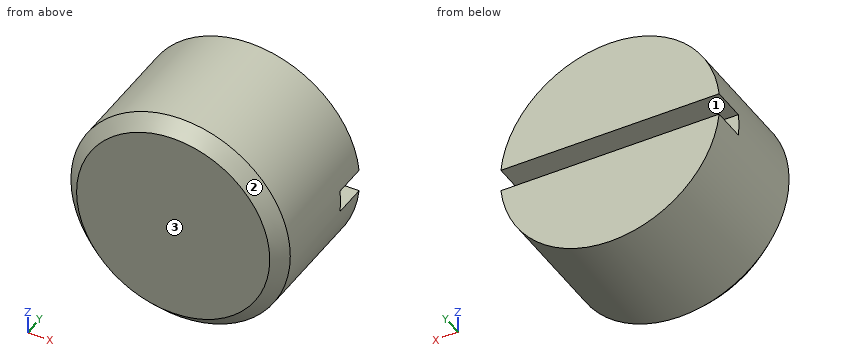
from build123d import *

# Parameters (mm, degrees)
SKETCH2_W          = 9.728
SKETCH2_H          = 1
CUT_EXTRUDE1_DEPTH = 1.5


with BuildPart() as part:
    # Sketch1 → Revolve1 (revolve)
    with BuildSketch(Plane.XY):
        Polygon((0, 0), (4.864, 0), (4.864, -5.419), (4.283, -6), (0, -6), align=None)
    revolve(axis=Axis((0, -6, 0), (0, 1, 0)))

    # Sketch2 → Cut-Extrude1 (cut)
    with BuildSketch(Plane(origin=(0, 0, 0), x_dir=(1, 0, 0), z_dir=(0, 1, 0))):
        Rectangle(SKETCH2_W, SKETCH2_H)
    extrude(amount=-CUT_EXTRUDE1_DEPTH, mode=Mode.SUBTRACT)


solid = part.part
Here's how the part is built. I have some questions about the finished solid (model axes, mm). Face numbers are marked on the shaded views. Coordinates: 2 decimals unless noted, no trailing zeros. Write each loop counter-clockwise with the first axis right and the second up, starting at its lowest first coordinate (ties: lowest second). Pieces come first, ordered by that corner, then holes. Notation, with made-up numbers: (-26.5, 52) - (-14.5, 52) arc R17 cw to (-14.5, 71) - close; hole circle Ø4 at (-1, 62.25). An arc over 180 degrees is marked (long way). Use one line per item in the form item = value.
1) Suppose I cut it at D-D, the plane y = -5. Write out the boundary of the cut face in (x, z).
Solved:
outline = circle Ø9.73 at (0, 0)
2) Thinking about a two-plate mould opening in Z: for the marked faces 1, 2 and 3, which applies, released by +Z, released by -Z, zero draft, split by the parting line, or undercut?
Solved:
face_1 = undercut
face_2 = split by the parting line
face_3 = zero draft
3) I'm going to push flat-ended pins straight in: P1, Ø2, axis at x = 3.5, y = -1.5, coming from the +Z side; P2, Ø1, axis at y = -5, z = -2, coming from the +X side; P3, Ø2, axis at y = -4.5, z = -2, coming from the -X side. Where does each tip first touch, or does it pass through?
Solved:
P1 = 4.17
P2 = 4.63
P3 = -4.76
4) I need wall thicknesses on line 1 (Z direction, x = 0.5, y = -0.7); line 2 (Z direction, x = -0.5, y = -4.5); line 3 (Z direction, x = -1.5, y = -1.1). Which ranges of each line are inside material? Lowest first, please.
Solved:
line_1 = -4.84 to -0.5, 0.5 to 4.84
line_2 = -4.84 to 4.84
line_3 = -4.63 to -0.5, 0.5 to 4.63
5) Suppose I cut it at A-A, the plane x = 0. Write out the boundary of the cut face in (y, z), plus the area to 3 significant figures.
Solved:
outline = (-6, -4.28) - (-5.42, -4.86) - (0, -4.86) - (0, -0.5) - (-1.5, -0.5) - (-1.5, 0.5) - (0, 0.5) - (0, 4.86) - (-5.42, 4.86) - (-6, 4.28) - close
area = 56.5 mm2
6) Suppose I cut it at C-C, the plane z = 0. Write out the boundary of the cut face in (x, y), plus the area to 3 significant figures.
Solved:
outline = (-4.86, -5.42) - (-4.28, -6) - (4.28, -6) - (4.86, -5.42) - (4.86, -1.5) - (-4.86, -1.5) - close
area = 43.4 mm2
